Could you check a few things on this model? Use its own coordinates, in mm. A direction names the side the tool comes from. Round coordinates to 2 decimals unless told otherwise and drop trailing zeros. Loops run counter-clockwise (first coordinate to the right, second up) from the corner with the lowest first, then second, coordinate; pieces in that order, holes last.
from build123d import *

# Parameters (mm, degrees)
F0_W          = 32
F0_H          = 32
F1_DEPTH      = 17
F2_R          = 8.05
F3_DEPTH      = 13
F3_DEPTH_BACK = 17
F4_W          = 32
F4_H          = 2
F5_DEPTH      = 16.001
F5_DEPTH_BACK = 16.001
F6_R          = 3.175
F6_R_2        = 2.5796875
F7_DEPTH      = 16.001
F7_DEPTH_BACK = 16.001
F8_R          = 1.625
F9_DEPTH      = 32.0010001
F10_R         = 3.55
F12_DEPTH     = 5.5
F13_DEPTH     = 10
F15_DEPTH     = 4.001
F16_W         = 9.5
F16_H         = 18


with BuildPart() as f1:
    # F0 (on Front) → F1 (new body, symmetric)
    with BuildSketch(Plane.XZ):
        Rectangle(F0_W, F0_H)
    extrude(amount=F1_DEPTH, both=True)

    # F2 (on Front) → F3 (cut, two sides)
    with BuildSketch(Plane.XZ) as f3_sk:
        Circle(F2_R)
    extrude(amount=-F3_DEPTH, mode=Mode.SUBTRACT)
    extrude(f3_sk.sketch, amount=F3_DEPTH_BACK, mode=Mode.SUBTRACT)

    # F4 (on Right) → F5 (cut, two sides)
    with BuildSketch(Plane.YZ) as f5_sk:
        with Locations((-3, 0)):
            Rectangle(F4_W, F4_H)
    extrude(amount=-F5_DEPTH, mode=Mode.SUBTRACT)
    extrude(f5_sk.sketch, amount=F5_DEPTH_BACK, mode=Mode.SUBTRACT)

    # F6 (on Top) → F7 (cut, two sides)
    with BuildSketch(Plane.XY) as f7_sk:
        with Locations((0, 6)):
            Circle(F6_R)
        with Locations((0, -4)):
            Circle(F6_R_2)
        with Locations((0, -13)):
            Circle(F6_R)
    extrude(amount=-F7_DEPTH, mode=Mode.SUBTRACT)
    extrude(f7_sk.sketch, amount=F7_DEPTH_BACK, mode=Mode.SUBTRACT)

    # F8 (on face) → F9 (cut, through all)
    with BuildSketch(Plane.XY.offset(16)):
        with Locations((-11, -12)):
            Circle(F8_R)
        with Locations((11, -12)):
            Circle(F8_R)
    extrude(amount=-F9_DEPTH, mode=Mode.SUBTRACT)

    # F10 (on face) → F12 (cut)
    with BuildSketch(Plane(origin=(0, 0, -16), x_dir=(1, 0, 0), z_dir=(0, 0, -1))):
        with Locations((11, 12)):
            Circle(F10_R)
        with Locations((-11, 12)):
            Circle(F10_R)
    extrude(amount=-F12_DEPTH, mode=Mode.SUBTRACT)

    # F11 (on face) → F13 (cut)
    with BuildSketch(Plane.XY.offset(16)):
        Polygon((-8, -13.7320508076), (-8, -10.2679491924), (-11, -8.5358983849), (-14, -10.2679491924), (-14, -13.7320508076), (-11, -15.4641016151), align=None)
        Polygon((8, -10.2679491924), (8, -13.7320508076), (11, -15.4641016151), (14, -13.7320508076), (14, -10.2679491924), (11, -8.5358983849), align=None)
    extrude(amount=-F13_DEPTH, mode=Mode.SUBTRACT)

    # F14 (on face) → F15 (cut, through all)
    with BuildSketch(Plane.XZ.offset(-13)):
        Polygon((0, -7.0710678119), (7.0710678119, 0), (0, 7.0710678119), (-7.0710678119, 0), align=None)
    extrude(amount=-F15_DEPTH, mode=Mode.SUBTRACT)

    # F16 (on Top) → F17 (revolve, cut)
    with BuildSketch(Plane.XY):
        with Locations((21.25, 3)):
            Rectangle(F16_W, F16_H)
    revolve(axis=Axis((0, -3.4330706112, 0), (0, -1, 0)), mode=Mode.SUBTRACT)


solid = f1.part
Item 1: If we section it at C-C, the plane y = -4: Please give me the cut outline in (x, z), then the cut area to 3 significant figures.
Results list:
outline: (-16, -4.03) arc R16.5 ccw to (-4.03, -16) - (-2.58, -16) - (-2.58, -7.63) arc R8.05 cw to (-7.99, -1) - (-16, -1) - close; (-16, 1) - (-7.99, 1) arc R8.05 cw to (-2.58, 7.63) - (-2.58, 16) - (-4.03, 16) arc R16.5 ccw to (-16, 4.03) - close; (2.58, -16) - (4.03, -16) arc R16.5 ccw to (16, -4.03) - (16, -1) - (7.99, -1) arc R8.05 cw to (2.58, -7.63) - close; (2.58, 7.63) arc R8.05 cw to (7.99, 1) - (16, 1) - (16, 4.03) arc R16.5 ccw to (4.03, 16) - (2.58, 16) - close
area: 526 mm2
Item 2: Will these pins go through, and if not, where does the flat tip stop? pin 1 (8.5 mm diameter, centred on x = 0, y = -4, fed in from +Z); pin 2 (2 mm diameter, centred on x = -10.5, y = 3, fed in from -Z); pin 3 (2 mm diameter, centred on y = 3.5, z = -10, fed in from +X); pin 4 (3.5 mm diameter, centred on x = -11, y = -12.5, fed in from -Z).
Results list:
pin 1: stops at z = 16
pin 2: stops at z = -13.49
pin 3: stops at x = 13.83
pin 4: stops at z = -10.5
Item 3: If we section it at B-B, the plane x = 12: Count the separate pieces of the cut face and the enclosed holes in it, then the cut area to 3 significant figures.
Results list:
separate pieces: 3
enclosed holes: 0
area: 727 mm2
Item 4: If we section it at D-D, the plane z = -6.5: Please give me the cut outline in (x, y) (3 decimals).
Results list:
outline: (-16, -17) - (-4.749, -17) - (-4.749, 13) - (-0.571, 13) - (-0.571, 17) - (-16, 17) - (-16, 12) - (-15.166, 12) - (-15.166, -6) - (-16, -6) - close; (0.571, 13) - (4.749, 13) - (4.749, -17) - (16, -17) - (16, -6) - (15.166, -6) - (15.166, 12) - (16, 12) - (16, 17) - (0.571, 17) - close; hole circle Ø3.25 at (-11, -12); hole circle Ø3.25 at (11, -12)
Item 5: If I drill on line 1 along Y through (x, z) = (0, -10) (3 decimals); line 2 along Y through (x, z) = (-11, -5.5) (3 decimals); line 3 along Y through (x, z) = (14, -9), over which ranges is the centre line in solid material (lowest first)?
Results list:
line 1: y = -17 to -16.175, -9.825 to -6.58, -1.42 to 2.825, 9.175 to 17
line 2: y = -17 to -13.625, -10.375 to 17
line 3: y = -17 to -6, 12 to 17
Item 6: For faces 4 (the flat face through (12, -10, -10.5)), 5 (the flat face through (3.585, 14.972, 3.486)), 6 (the flat face through (-14, -12, 11)), 7 (the flat face through (-13, 12, -13)), which set-ups out of +Z, -Z, +X, -X, +Y, -Y let a thin tool reach every point of the face, with its end or its side?
Results list:
face 4: -Z
face 5: +Y, -Y
face 6: +Z
face 7: -Z, -X
Item 7: If we section it at A-A, the plane y = 11.5: Please give me the cut outline in (x, z), then the cut area to 3 significant figures.
Results list:
outline: (-16, -4.03) arc R16.5 ccw to (-4.03, -16) - (4.03, -16) arc R16.5 ccw to (16, -4.03) - (16, -1) - (7.99, -1) arc R8.05 cw to (-7.99, -1) - (-16, -1) - close; (-16, 1) - (-7.99, 1) arc R8.05 cw to (7.99, 1) - (16, 1) - (16, 4.03) arc R16.5 ccw to (4.03, 16) - (-4.03, 16) arc R16.5 ccw to (-16, 4.03) - close
area: 609 mm2
Item 8: We'd pull the mould along Y, two halves only. Please class faces 1 (the flat face through (0, -17, -10)), 2 (the cylindrical face through (-7.614, -13.066, -13.288)), 3 (the flat face through (-3.486, 14.972, 3.585)): released by +Y, released by -Y, zero draft, split by the parting line, or undercut.
Results list:
face 1: released by -Y
face 2: undercut
face 3: zero draft
